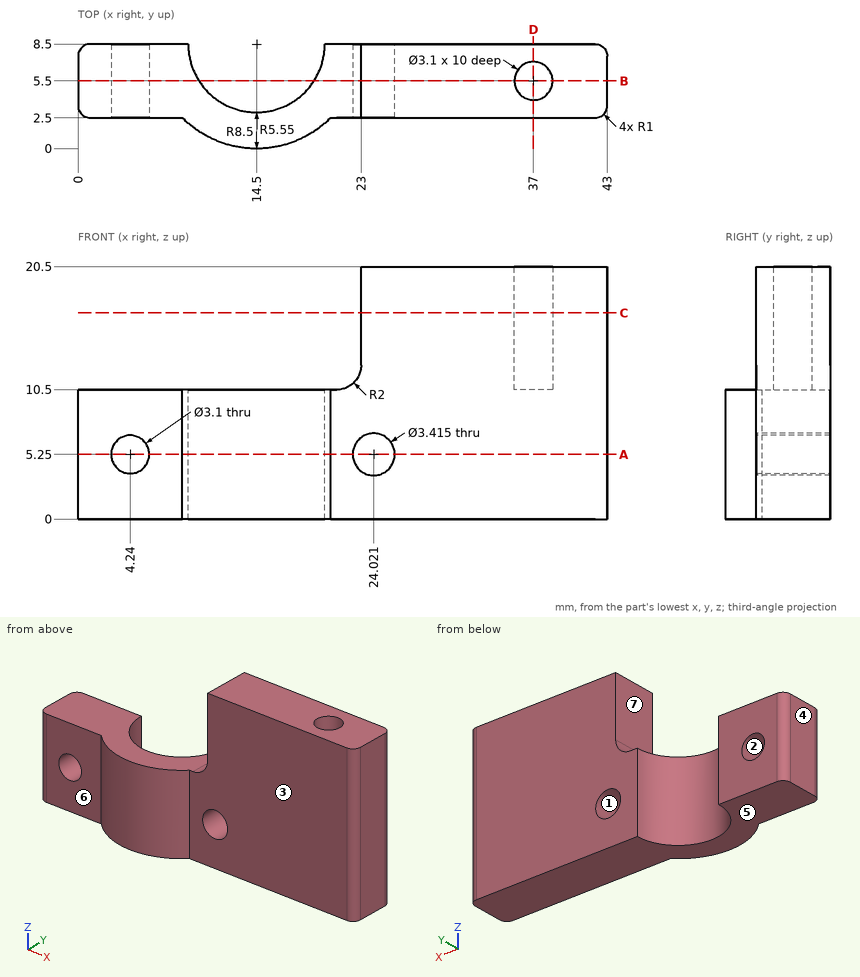
The figure shows three views and two pictorial views of one solid part (mm, origin at its lowest corner). Answer the questions. A direction names the side the tool comes from. Coordinates: 2 decimals unless noted, no trailing zeros. Order: outer loops, then holes, each group sorted by start corner. A loop starts at its lowest first (then second) coordinate and runs counter-clockwise, first axis right, second up.
Q1. A cutting plane is placed at C-C, the plane z = 16.75. Write down the section's boundary in (x, y), and give its area (3 significant figures).
Q2. Given P1, Ø6, axis at x = 28, z = 8, coming from the -Y side; P2, Ø3, axis at x = 24.02, z = 5.25, coming from the +Y side; P3, Ø1.8, axis at y = 4, z = 14.5, coming from the -X side; P4, Ø2.5, axis at x = 10.5, y = 3, coming from the +Z side, each flat-ended and moving along its own axis, determine where each tip first touches the part or whether it passes through.
Q3. A cutting plane is placed at D-D, the plane x = 37. Write down the section's boundary in (y, z).
Q4. For a pull along X with two mould halves and no side action, classify the marked faces 1, 2, 3 and 4 as pulls with the +X half, pulls with the -X half, needs draft (parallel to the pull), parting line crosses it, or undercut.
Q5. A cutting plane is placed at A-A, the plane z = 5.25. Write down the section's boundary in (x, y).
Q6. Consider line 1 (X direction, y = 5.5, z = 6.5) (1 decimal); line 2 (Z direction, x = 19.5, y = 6); line 3 (Y direction, x = 27.5, z = 2.75). Determine where each line is inside the solid, lowest interval first.
Q7. A cutting plane is placed at B-B, the plane y = 5.5. State how many separate pieces and enclosed holes the cut face has.
Q8. Which of the six approach directions +Z, -Z, +X, -X, +Y, -Y give full straight-line access (tool end or side, diameter ignored) to the marked faces 5, 6 and 7?
Answers follow:
1. outline: (23, 2.5) - (42, 2.5) arc R1 ccw to (43, 3.5) - (43, 7.5) arc R1 ccw to (42, 8.5) - (23, 8.5) - close; hole circle Ø3.1 at (37, 5.5)
1. area: 112 mm2
2. P1: stops at y = 2.5
2. P2: passes through
2. P3: stops at x = 23
2. P4: stops at z = 10.5
3. outline: (2.5, 0) - (8.5, 0) - (8.5, 20.5) - (7.05, 20.5) - (7.05, 10.5) - (3.95, 10.5) - (3.95, 20.5) - (2.5, 20.5) - close
4. face 1: undercut
4. face 2: undercut
4. face 3: needs draft
4. face 4: pulls with the -X half
5. outline: (0, 3.5) arc R1 ccw to (1, 2.5) - (2.69, 2.5) - (2.69, 8.5) - (1, 8.5) arc R1 ccw to (0, 7.5) - close; (5.79, 2.5) - (8.48, 2.5) arc R8.5 ccw to (20.52, 2.5) - (22.31, 2.5) - (22.31, 8.5) - (20.05, 8.5) arc R5.55 cw to (8.95, 8.5) - (5.79, 8.5) - close; (25.73, 2.5) - (42, 2.5) arc R1 ccw to (43, 3.5) - (43, 7.5) arc R1 ccw to (42, 8.5) - (25.73, 8.5) - close
6. line 1: x = 0 to 3.3, 5.2 to 9.8, 19.2 to 22.9, 25.2 to 43
6. line 2: z = 0 to 10.5
6. line 3: y = 2.5 to 8.5
7. separate pieces: 2
7. enclosed holes: 2
8. face 5: -Z, +X, -X, +Y, -Y
8. face 6: +Z, -Z, -X, -Y
8. face 7: +Z, -X, +Y, -Y
